Part model, mm, in its own coordinate system. Face numbers are marked on the shaded views. A direction names the side the tool comes from. Round coordinates to 2 decimals unless told otherwise and drop trailing zeros. Order: outer loops, then holes, each group sorted by start corner. A loop starts at its lowest first (then second) coordinate and runs counter-clockwise, first axis right, second up. Notation, with made-up numbers: (32, 65) - (54, 65) arc R16 ccw to (54, 76) - close; hole circle Ø2 at (-13.5, 59.25). An arc over 180 degrees is marked (long way). Return JSON: item names as keys, results as strings. Group by question number.
Item 1: Drop flat-ended pins along their axis: pin 1 (2 mm diameter, centred on x = 2, y = -0.5, fed in from +Z); pin 2 (0.7 mm diameter, centred on y = 0, z = 0, fed in from -X); pin 3 (1 mm diameter, centred on y = 0, z = -1.5, fed in from +X); pin 4 (2 mm diameter, centred on x = 6, z = -1, fed in from +Y). Give the stop position or say it passes through.
Item 2: Tool access for the marked faces 3 and 4: list every direction of +Z, -Z, +X, -X, +Y, -Y with a clear straight run to the whole face (end or side of a thin tool).
Item 3: Probe probe 1 along X at (y, z) = (-0.1, 1.95); probe 2 along Z at (x, y) = (3.5, -0.5); probe 3 along X at (y, z) = (1.15, 0.9). List the from-to ranges inside material, lowest first.
Item 4: Saw through at A-A on x = 3.25. List the corners of the cut face in (y, z).
Item 5: Two-plate mould, pull along Y, no slides. Class the marked faces 1 and 2: released by +Y, released by -Y, zero draft, split by the parting line, or undercut.
Item 6: Saw through at B-B on x = 2. List the corners of the cut face in (y, z), and give its area (3 significant figures).
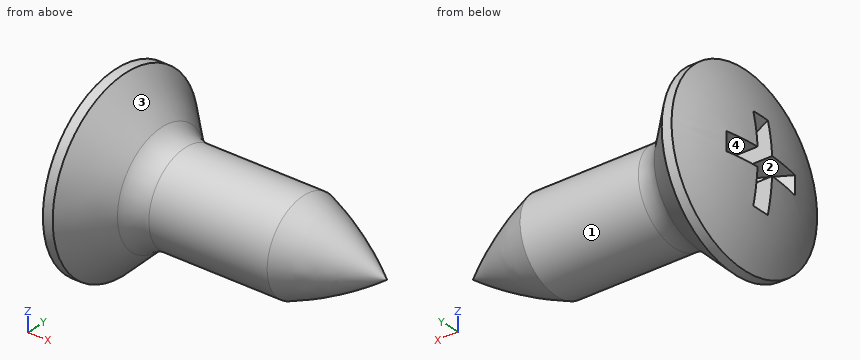
```python
from build123d import *

# Parameters (mm, degrees)
CROSSRECESS_DEPTH = 1.2
DRAFT1_ANGLE      = -30


with BuildPart() as part:
    # Sketch1 → Base (revolve)
    with BuildSketch(Plane.XY):
        with BuildLine():
            Line((7, 0), (7, 1.1))
            Line((7, 1.1), (2.165685425, 1.1))
            ThreePointArc((2.165685425, 1.1), (1.859538679, 1.160896374), (1.6, 1.334314575))
            Line((1.6, 1.334314575), (0.734314575, 2.2))
            Line((0.734314575, 2.2), (0.5, 2.2))
            ThreePointArc((0.5, 2.2), (0.126573764, 1.128051417), (0, 0))
            Line((0, 0), (7, 0))
        make_face()
    revolve(axis=Axis((-20.418228315, 0, 0), (1, 0, 0)))

    # Sketch2 → CrossRecess (cut)
    with BuildSketch(Plane(origin=(0, 0, 0), x_dir=(0, 0, -1), z_dir=(1, 0, 0))):
        Polygon((-0.22, 1.1), (0.22, 1.1), (0.22, 0.22), (1.1, 0.22), (1.1, -0.22), (0.22, -0.22), (0.22, -1.1), (-0.22, -1.1), (-0.22, -0.22), (-1.1, -0.22), (-1.1, 0.22), (-0.22, 0.22), align=None)
    extrude(amount=CROSSRECESS_DEPTH, mode=Mode.SUBTRACT)

    # Sketch5 → Cut-Revolve6 (revolve, cut)
    with BuildSketch(Plane.XY):
        with BuildLine():
            Line((7, 0), (7.5, 0))
            Line((7.5, 0), (7.5, -1.1))
            Line((7.5, -1.1), (7, -1.1))
            Line((7, -1.1), (5, -1.1))
            ThreePointArc((5, -1.1), (6.03943286, -0.621696108), (7, 0))
        make_face()
    revolve(axis=Axis((37.040663239, 0, 0), (-1, 0, 0)), mode=Mode.SUBTRACT)

    # Draft1
    draft1_faces = [part.faces().sort_by_distance(p)[0] for p in [
        (0.660951691, -1.1, 0),
        (0.660951691, 0, -1.1),
        (0.660951691, 0, 1.1),
        (0.660951691, 1.1, 0),
    ]]
    draft(draft1_faces, Plane(origin=(0, 0, 0), x_dir=(0, 0, 1), z_dir=(1, 0, 0)), DRAFT1_ANGLE)


solid = part.part
```
Filled in:
{
 "1": {"pin 1": "stops at z = 1.89", "pin 2": "stops at x = 0.01", "pin 3": "stops at x = 5.25", "pin 4": "stops at y = 0.94"},
 "2": {"face 3": "+X", "face 4": "-X"},
 "3": {"probe 1": "x = 0.39 to 0.98", "probe 2": "z = -0.98 to 0.98", "probe 3": "x = 0.21 to 1.47"},
 "4": {"outline": "circle Ø2.2 at (0, 0)"},
 "5": {"face 1": "split by the parting line", "face 2": "undercut"},
 "6": {"outline": "circle Ø2.23 at (0, 0)", "area": "3.92 mm^2"}
}
